```python
from build123d import *

# Parameters (mm, degrees)
F0_W      = 139.3444
F0_H      = 139.3444
F1_DEPTH  = 165.1
F3_W      = 139.3444
F3_H      = 139.3444
F3_R      = 66.04
F4_DEPTH  = 114.3
F5_R      = 63.5
F6_DEPTH  = 165.101
F7_R      = 63.5
F8_DEPTH  = 2.54
F9_R      = 63.5
F10_DEPTH = 6.35
F11_R     = 12.7
F12_DEPTH = 63.5
F13_W     = 215.9
F13_H     = 165.1
F14_DEPTH = 3.81
F16_D     = 13.1064
F17_R     = 63.5
F17_R_2   = 12.7
F18_DEPTH = 2.54


with BuildPart() as f1:
    # F0 (on Front) → F1 (new body)
    with BuildSketch(Plane.XZ):
        Rectangle(F0_W, F0_H)
    extrude(amount=F1_DEPTH)

    # F3 (on offset) → F4 (cut)
    with BuildSketch(Plane.XZ.offset(139.7)):
        Rectangle(F3_W, F3_H)
        Circle(F3_R, mode=Mode.SUBTRACT)
    extrude(amount=-F4_DEPTH, mode=Mode.SUBTRACT)

    # F5 (on face) → F6 (cut, through all)
    with BuildSketch(Plane.XZ.offset(165.1)):
        Circle(F5_R)
    extrude(amount=-F6_DEPTH, mode=Mode.SUBTRACT)

    # F7 (on face) → F8 (join)
    with BuildSketch(Plane(origin=(0, 0, 0), x_dir=(-1, 0, 0), z_dir=(0, 1, 0))):
        Circle(F7_R)
    extrude(amount=-F8_DEPTH)

    # F9 (on offset) → F10 (join)
    with BuildSketch(Plane.XZ.offset(139.7)):
        Circle(F9_R)
    extrude(amount=F10_DEPTH)

    # F11 (on face) → F12 (join)
    with BuildSketch(Plane.XZ.offset(146.05)):
        Circle(F11_R)
    extrude(amount=F12_DEPTH)

    # F13 (on face) → F14 (join)
    with BuildSketch(Plane(origin=(0, 0, 0), x_dir=(-1, 0, 0), z_dir=(0, 1, 0))):
        Rectangle(F13_W, F13_H)
    extrude(amount=F14_DEPTH)

    # F16 (through all)
    with Locations(Plane.XZ):
        with Locations((91.44, 64.77), (91.44, -64.77), (-91.44, 64.77), (-91.44, -64.77)):
            Hole(F16_D / 2)

    # F17 (on face) → F18 (join)
    with BuildSketch(Plane.XZ.offset(165.1)):
        Circle(F17_R)
        Circle(F17_R_2, mode=Mode.SUBTRACT)
    extrude(amount=-F18_DEPTH)


solid = f1.part
```
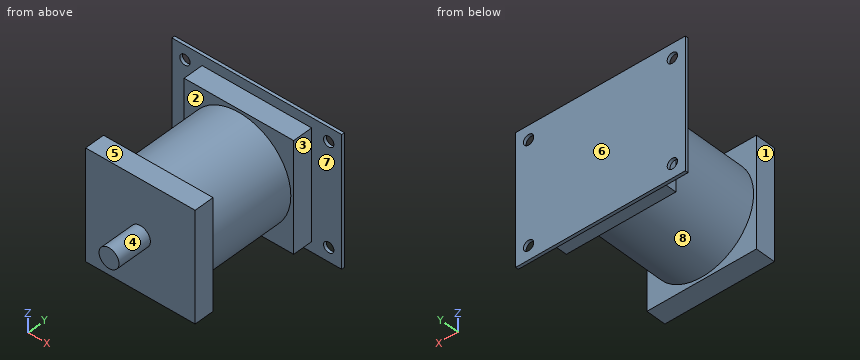
Source: CAD feature listing. Evaluate the final solid. Frame: model axes, mm. Face numbers are marked on the shaded views. A direction names the side the tool comes from. Round coordinates to 2 decimals unless told otherwise and drop trailing zeros. Loops run counter-clockwise (first coordinate to the right, second up) from the corner with the lowest first, then second, coordinate; pieces in that order, holes last. Notation, with made-up numbers: (51.5, 2.5) - (91.5, 2.5) arc R19 ccw to (91.5, 13.5) - close; hole circle Ø3 at (-33, 56.25). An arc over 180 degrees is marked (long way). Use CSV: the item, a comma, the result in double quotes.
Q1. Section query A-A, the plane x = -91.44. Output: boundary loops of the cut face in (y, z), then the cut area to 3 significant figures.
Reported:
outline,"(0, -82.55) - (3.81, -82.55) - (3.81, -71.32) - (0, -71.32) - close; (0, -58.22) - (3.81, -58.22) - (3.81, 58.22) - (0, 58.22) - close; (0, 71.32) - (3.81, 71.32) - (3.81, 82.55) - (0, 82.55) - close"
area,"529 mm^2"
Q2. Reachability of the marked faces 1, 2, 3 and 4 from +Z, -Z, +X, -X, +Y, -Y: full face, straight path, thin tool, end or side. Return the list, or none.
Reported:
face 1,"+Z, -Z, -X, -Y"
face 2,"none"
face 3,"+Z, -Z, +X, -Y"
face 4,"-Y"
Q3. Pin query (flat end, axial travel): pin 1 Ø4 at (x, y) = (14, -108.5) entering from -Z; pin 2 Ø1.5 at (y, z) = (-29, -7) entering from +X; pin 3 Ø20.5 at (x, y) = (-23, -156.5) entering from -Z. Return the tip coordinate at first contact, or that it passes through.
Reported:
pin 1,"z = -64.94"
pin 2,"x = 65.74"
pin 3,"z = -69.67"
Q4. Ray query, line 1 along Y through (x, z) = (50.5, -12.5); line 2 along X through (y, z) = (2, 64); line 3 along Z through (x, y) = (91.44, 1.3). Return the intervals inside material, ascending.
Reported:
line 1,"-165.1 to -162.56, -146.05 to -139.7, -2.54 to 3.81"
line 2,"-107.95 to -97.95, -84.93 to 84.93, 97.95 to 107.95"
line 3,"-82.55 to -71.32, -58.22 to 58.22, 71.32 to 82.55"
Q5. Section query D-D, the plane z = 23.5. Output: boundary loops of the cut face in (x, y), then the cut area to 3 significant figures.
Reported:
outline,"(-107.95, 0) - (-69.67, 0) - (-69.67, -25.4) - (-61.72, -25.4) - (-61.72, -139.7) - (-69.67, -139.7) - (-69.67, -165.1) - (69.67, -165.1) - (69.67, -139.7) - (61.72, -139.7) - (61.72, -25.4) - (69.67, -25.4) - (69.67, 0) - (107.95, 0) - (107.95, 3.81) - (-107.95, 3.81) - close; hole (-58.99, -162.56) - (58.99, -162.56) - (58.99, -146.05) - (-58.99, -146.05) - close; hole (-58.99, -139.7) - (58.99, -139.7) - (58.99, -2.54) - (-58.99, -2.54) - close"
area,"3,880 mm^2"
Q6. Section query C-C, the plane z = 0. Give the number of separate pieces and of enclosed holes in the cut face, then the cut area to 3 significant figures.
Reported:
separate pieces,"1"
enclosed holes,"3"
area,"5,030 mm^2"
Q7. Section query B-B, the plane y = -151. Output: boundary loops of the cut face in (x, z), then the cut area to 3 significant figures.
Reported:
outline,"(-69.67, -69.67) - (69.67, -69.67) - (69.67, 69.67) - (-69.67, 69.67) - close; circle Ø25.4 at (0, 0); hole circle Ø127 at (0, 0)"
area,"7,260 mm^2"
Q8. Mould query, pull axis Y, two halves, no side actions, for the marked faces 5, 6, 7 and 8. Classes: pulls with the +Y half, pulls with the -Y half, needs draft (parallel to the pull), parting line crosses it, or undercut.
Reported:
face 5,"needs draft"
face 6,"pulls with the +Y half"
face 7,"pulls with the -Y half"
face 8,"undercut"
